Design review of the part built by this model. Coordinates are the model's own, in mm. A direction names the side the tool comes from. Give positions to 0.01 mm unless a question says otherwise; leave off trailing zeros. Write each loop counter-clockwise with the first axis right and the second up, starting at its lowest first coordinate (ties: lowest second). Pieces come first, ordered by that corner, then holes. Notation, with made-up numbers: M 39,-0.75 L 59,-0.75 A13 ccw 59,16.25 Z; hole C 41.25,76.5 d3. An arc over 180 degrees is marked long. Use one line per item in the form item = value. Start each with the question number.
from build123d import *

# Parameters (mm, degrees)
SKETCH1_R           = 22.45
SKETCH1_R_2         = 18.55
SKETCH1_R_3         = 6.11
SKETCH1_R_4         = 5.25
SKETCH1_R_5         = 3.075
BOSS_EXTRUDE1_DEPTH = 5.5
SKETCH1_3_R         = 22.45
SKETCH1_3_R_2       = 18.55
SKETCH1_3_R_3       = 6.11
BOSS_EXTRUDE2_DEPTH = 6
SKETCH1_4_R         = 22.45
SKETCH1_4_R_2       = 18.55
BOSS_EXTRUDE3_DEPTH = 17
BOSS_EXTRUDE4_DEPTH = 10
DRAFT1_ANGLE        = 45
BOSS_EXTRUDE5_DEPTH = 3
SKETCH4_R           = 3.075
BOSS_EXTRUDE6_DEPTH = 1.5
SKETCH3_R           = 1.5
SKETCH3_R_2         = 1.55
CUT_EXTRUDE1_DEPTH  = 11
CUT_EXTRUDE2_START  = -9.6
SKETCH3_4_R         = 1.5
CUT_EXTRUDE2_DEPTH  = 2.6
CUT_EXTRUDE3_START  = -8
SKETCH3_5_R         = 1.55
CUT_EXTRUDE3_DEPTH  = 2.5


with BuildPart() as part:
    # Sketch1 → Boss-Extrude1 (new body)
    with BuildSketch(Plane.ZY.offset(-4.58817912)):
        with BuildLine():
            Line((173.913255387, 21.29653024), (97.713255387, 21.29653024))
            Line((97.713255387, 21.29653024), (97.713255387, 24.29653024))
            Line((97.713255387, 24.29653024), (94.713255387, 24.29653024))
            Line((94.713255387, 24.29653024), (94.713255387, 18.29653024))
            ThreePointArc((94.713255387, 18.29653024), (95.445488434, 16.528763287), (97.213255387, 15.79653024))
            Line((97.213255387, 15.79653024), (102.52576333, 15.79653024))
            Line((102.52576333, 15.79653024), (102.52576333, -6.35346976))
            ThreePointArc((102.52576333, -6.35346976), (124.97576333, 16.09653024), (147.42576333, -6.35346976))
            Line((147.42576333, -6.35346976), (147.42576333, 13.29653024))
            Line((147.42576333, 13.29653024), (171.913255387, 13.29653024))
            ThreePointArc((171.913255387, 13.29653024), (175.448789293, 14.760996334), (176.913255387, 18.29653024))
            Line((176.913255387, 18.29653024), (176.913255387, 24.29653024))
            Line((176.913255387, 24.29653024), (173.913255387, 24.29653024))
            Line((173.913255387, 24.29653024), (173.913255387, 21.29653024))
        make_face()
        with BuildLine():
            ThreePointArc((124.97576333, -28.80346976), (109.101216092, -22.228016998), (102.52576333, -6.35346976))
            Line((102.52576333, -6.35346976), (102.52576333, -28.80346976))
            Line((102.52576333, -28.80346976), (124.97576333, -28.80346976))
        make_face()
        with Locations((124.97576333, -6.35346976)):
            Circle(SKETCH1_R)
        with Locations((124.97576333, -6.35346976)):
            Circle(SKETCH1_R_2, mode=Mode.SUBTRACT)
        with Locations((124.97576333, -6.35346976)):
            Circle(SKETCH1_R_2)
        with Locations((131.813255387, -4.853902367)):
            Circle(SKETCH1_R_3, mode=Mode.SUBTRACT)
        with Locations((131.813255387, -4.853902367)):
            Circle(SKETCH1_R_3)
        with Locations((131.813255387, -4.853902367)):
            Circle(SKETCH1_R_4, mode=Mode.SUBTRACT)
        with Locations((131.813255387, -4.853902367)):
            Circle(SKETCH1_R_4)
        with Locations((131.813255387, -4.853902367)):
            Circle(SKETCH1_R_5, mode=Mode.SUBTRACT)
        with BuildLine():
            Line((147.42576333, -28.80346976), (147.42576333, -6.35346976))
            ThreePointArc((147.42576333, -6.35346976), (140.850310568, -22.228016998), (124.97576333, -28.80346976))
            Line((124.97576333, -28.80346976), (147.42576333, -28.80346976))
        make_face()
    extrude(amount=BOSS_EXTRUDE1_DEPTH)

    # Sketch1<3> → Boss-Extrude2 (add)
    with BuildSketch(Plane.ZY.offset(-4.58817912)):
        with BuildLine():
            Line((173.913255387, 21.29653024), (97.713255387, 21.29653024))
            Line((97.713255387, 21.29653024), (97.713255387, 24.29653024))
            Line((97.713255387, 24.29653024), (94.713255387, 24.29653024))
            Line((94.713255387, 24.29653024), (94.713255387, 18.29653024))
            ThreePointArc((94.713255387, 18.29653024), (95.445488434, 16.528763287), (97.213255387, 15.79653024))
            Line((97.213255387, 15.79653024), (102.52576333, 15.79653024))
            Line((102.52576333, 15.79653024), (102.52576333, -6.35346976))
            ThreePointArc((102.52576333, -6.35346976), (124.97576333, 16.09653024), (147.42576333, -6.35346976))
            Line((147.42576333, -6.35346976), (147.42576333, 13.29653024))
            Line((147.42576333, 13.29653024), (171.913255387, 13.29653024))
            ThreePointArc((171.913255387, 13.29653024), (175.448789293, 14.760996334), (176.913255387, 18.29653024))
            Line((176.913255387, 18.29653024), (176.913255387, 24.29653024))
            Line((176.913255387, 24.29653024), (173.913255387, 24.29653024))
            Line((173.913255387, 24.29653024), (173.913255387, 21.29653024))
        make_face()
        with BuildLine():
            Line((147.42576333, -28.80346976), (147.42576333, -6.35346976))
            ThreePointArc((147.42576333, -6.35346976), (140.850310568, -22.228016998), (124.97576333, -28.80346976))
            Line((124.97576333, -28.80346976), (147.42576333, -28.80346976))
        make_face()
        with Locations((124.97576333, -6.35346976)):
            Circle(SKETCH1_3_R)
        with Locations((124.97576333, -6.35346976)):
            Circle(SKETCH1_3_R_2, mode=Mode.SUBTRACT)
        with Locations((124.97576333, -6.35346976)):
            Circle(SKETCH1_3_R_2)
        with Locations((131.813255387, -4.853902367)):
            Circle(SKETCH1_3_R_3, mode=Mode.SUBTRACT)
    extrude(amount=-BOSS_EXTRUDE2_DEPTH)

    # Sketch1<4> → Boss-Extrude3 (add)
    with BuildSketch(Plane.ZY.offset(-4.58817912)):
        with BuildLine():
            Line((173.913255387, 21.29653024), (97.713255387, 21.29653024))
            Line((97.713255387, 21.29653024), (97.713255387, 24.29653024))
            Line((97.713255387, 24.29653024), (94.713255387, 24.29653024))
            Line((94.713255387, 24.29653024), (94.713255387, 18.29653024))
            ThreePointArc((94.713255387, 18.29653024), (95.445488434, 16.528763287), (97.213255387, 15.79653024))
            Line((97.213255387, 15.79653024), (102.52576333, 15.79653024))
            Line((102.52576333, 15.79653024), (102.52576333, -6.35346976))
            ThreePointArc((102.52576333, -6.35346976), (124.97576333, 16.09653024), (147.42576333, -6.35346976))
            Line((147.42576333, -6.35346976), (147.42576333, 13.29653024))
            Line((147.42576333, 13.29653024), (171.913255387, 13.29653024))
            ThreePointArc((171.913255387, 13.29653024), (175.448789293, 14.760996334), (176.913255387, 18.29653024))
            Line((176.913255387, 18.29653024), (176.913255387, 24.29653024))
            Line((176.913255387, 24.29653024), (173.913255387, 24.29653024))
            Line((173.913255387, 24.29653024), (173.913255387, 21.29653024))
        make_face()
        with BuildLine():
            Line((147.42576333, -28.80346976), (147.42576333, -6.35346976))
            ThreePointArc((147.42576333, -6.35346976), (140.850310568, -22.228016998), (124.97576333, -28.80346976))
            Line((124.97576333, -28.80346976), (147.42576333, -28.80346976))
        make_face()
        with BuildLine():
            ThreePointArc((124.97576333, -28.80346976), (109.101216092, -22.228016998), (102.52576333, -6.35346976))
            Line((102.52576333, -6.35346976), (102.52576333, -28.80346976))
            Line((102.52576333, -28.80346976), (124.97576333, -28.80346976))
        make_face()
        with Locations((124.97576333, -6.35346976)):
            Circle(SKETCH1_4_R)
        with Locations((124.97576333, -6.35346976)):
            Circle(SKETCH1_4_R_2, mode=Mode.SUBTRACT)
    extrude(amount=-BOSS_EXTRUDE3_DEPTH)

    # Sketch2 → Boss-Extrude4 (add)
    with BuildSketch(Plane(origin=(21.58817912, 0, 0), x_dir=(0, 0, -1), z_dir=(1, 0, 0))):
        with BuildLine():
            Line((-151.941714705, 21.29653024), (-111.68479607, 21.29653024))
            ThreePointArc((-111.68479607, 21.29653024), (-131.813255387, 28.146097633), (-151.941714705, 21.29653024))
        make_face()
    extrude(amount=-BOSS_EXTRUDE4_DEPTH)

    # Draft1
    draft1_faces = [part.faces().sort_by_distance(p)[0] for p in [
        (11.58817912, 24.062292156, 131.813255387),
    ]]
    draft(draft1_faces, Plane(origin=(-98.771158707, 21.29653024, 0), x_dir=(1, 0, 0), z_dir=(0, 1, 0)), DRAFT1_ANGLE)

    # Sketch3<3> → Boss-Extrude5 (add)
    with BuildSketch(Plane(origin=(0, 21.29653024, 0), x_dir=(1, 0, 0), z_dir=(0, 1, 0))):
        with BuildLine():
            Line((-0.91182088, -173.913255387), (3.08817912, -173.913255387))
            ThreePointArc((3.08817912, -173.913255387), (0.526929425, -173.014817506), (-0.91182088, -170.713255387))
            Line((-0.91182088, -170.713255387), (-0.91182088, -173.913255387))
        make_face()
    extrude(amount=BOSS_EXTRUDE5_DEPTH)

    # Sketch4 → Boss-Extrude6 (add)
    with BuildSketch(Plane.ZY.offset(0.91182088)):
        with BuildLine():
            Line((97.713255387, 21.29653024), (97.713255387, 24.29653024))
            Line((97.713255387, 24.29653024), (94.713255387, 24.29653024))
            Line((94.713255387, 24.29653024), (94.713255387, 18.29653024))
            ThreePointArc((94.713255387, 18.29653024), (95.445488434, 16.528763287), (97.213255387, 15.79653024))
            Line((97.213255387, 15.79653024), (102.52576333, 15.79653024))
            Line((102.52576333, 15.79653024), (102.52576333, -28.80346976))
            Line((102.52576333, -28.80346976), (147.42576333, -28.80346976))
            Line((147.42576333, -28.80346976), (147.42576333, 13.29653024))
            Line((147.42576333, 13.29653024), (171.913255387, 13.29653024))
            ThreePointArc((171.913255387, 13.29653024), (175.448789293, 14.760996334), (176.913255387, 18.29653024))
            Line((176.913255387, 18.29653024), (176.913255387, 24.29653024))
            Line((176.913255387, 24.29653024), (170.713255387, 24.29653024))
            Line((170.713255387, 24.29653024), (170.713255387, 21.29653024))
            Line((170.713255387, 21.29653024), (155.075991135, 21.29653024))
            Line((155.075991135, 21.29653024), (108.550519639, 21.29653024))
            Line((108.550519639, 21.29653024), (97.713255387, 21.29653024))
        make_face()
        with Locations((131.813255387, -4.853902367)):
            Circle(SKETCH4_R, mode=Mode.SUBTRACT)
        with BuildLine():
            Line((112.44182594, 24.29653024), (97.713255387, 24.29653024))
            Line((97.713255387, 24.29653024), (97.713255387, 21.29653024))
            Line((97.713255387, 21.29653024), (108.550519639, 21.29653024))
            ThreePointArc((108.550519639, 21.29653024), (110.443463379, 22.864899727), (112.44182594, 24.29653024))
        make_face()
        with BuildLine():
            ThreePointArc((151.184684835, 24.29653024), (153.183047396, 22.864899727), (155.075991135, 21.29653024))
            Line((155.075991135, 21.29653024), (170.713255387, 21.29653024))
            Line((170.713255387, 21.29653024), (170.713255387, 24.29653024))
            Line((170.713255387, 24.29653024), (151.184684835, 24.29653024))
        make_face()
    extrude(amount=BOSS_EXTRUDE6_DEPTH)

    # Sketch3 → Cut-Extrude1 (cut)
    with BuildSketch(Plane(origin=(0, 21.29653024, 0), x_dir=(1, 0, 0), z_dir=(0, 1, 0))):
        with Locations(Location((2.879075654, -104.850755387, 0), (0, 0, 180))):
            Circle(SKETCH3_R)
        with Locations(Location((10.297282585, -104.850755387, 0), (0, 0, 180))):
            Circle(SKETCH3_R)
        with Locations(Location((3.11317912, -163.38083505, 0), (0, 0, 180))):
            Circle(SKETCH3_R_2)
    extrude(amount=-CUT_EXTRUDE1_DEPTH, mode=Mode.SUBTRACT)

    # Sketch3<4> → Cut-Extrude2 (cut)
    with BuildSketch(Plane(origin=(0, 21.29653024, 0), x_dir=(1, 0, 0), z_dir=(0, 1, 0)).offset(CUT_EXTRUDE2_START)):
        Polygon((7.447282585, -106.496203654), (10.297282585, -108.141651922), (13.147282585, -106.496203654), (13.147282585, -103.20530712), (11.970278215, -102.52576333), (8.624286956, -102.52576333), (7.447282585, -103.20530712), align=None)
        with Locations(Location((10.297282585, -104.850755387, 0), (0, 0, 180))):
            Circle(SKETCH3_4_R, mode=Mode.SUBTRACT)
        Polygon((11.970278215, -102.52576333), (13.147282585, -103.20530712), (13.147282585, -102.52576333), align=None)
        Polygon((7.447282585, -102.52576333), (7.447282585, -103.20530712), (8.624286956, -102.52576333), align=None)
        Polygon((0.029075654, -106.496203654), (2.879075654, -108.141651922), (5.729075654, -106.496203654), (5.729075654, -103.20530712), (4.552071284, -102.52576333), (1.206080025, -102.52576333), (0.029075654, -103.20530712), align=None)
        with Locations(Location((2.879075654, -104.850755387, 0), (0, 0, 180))):
            Circle(SKETCH3_4_R, mode=Mode.SUBTRACT)
        Polygon((4.552071284, -102.52576333), (5.729075654, -103.20530712), (5.729075654, -102.52576333), align=None)
        Polygon((0.029075654, -102.52576333), (0.029075654, -103.20530712), (1.206080025, -102.52576333), align=None)
    extrude(amount=CUT_EXTRUDE2_DEPTH, mode=Mode.SUBTRACT)

    # Sketch3<5> → Cut-Extrude3 (cut)
    with BuildSketch(Plane(origin=(0, 21.29653024, 0), x_dir=(1, 0, 0), z_dir=(0, 1, 0)).offset(CUT_EXTRUDE3_START)):
        Polygon((4.758627387, -160.53083505), (1.467730853, -160.53083505), (-0.177717415, -163.38083505), (1.467730853, -166.23083505), (4.758627387, -166.23083505), (6.404075654, -163.38083505), align=None)
        with Locations(Location((3.11317912, -163.38083505, 0), (0, 0, 180))):
            Circle(SKETCH3_5_R, mode=Mode.SUBTRACT)
    extrude(amount=CUT_EXTRUDE3_DEPTH, mode=Mode.SUBTRACT)


solid = part.part
1. We need section B-B (z = 168.5). State the section outline as (x, y) points.
2. Clearance check with flat-ended pins moving along their axes: pin 1 Ø2.5 at (x, z) = (9.5, 105.5) entering from +Y; pin 2 Ø2 at (x, y) = (17.5, -4.5) entering from -Z; pin 3 Ø18.5 at (y, z) = (-4.5, 123.5) entering from +X; pin 4 Ø2.5 at (y, z) = (22.5, 165.5) entering from +X. State where each tip first meets the part, or that it passes through.
3. To check wall thickness, follow L1, parallel to Y at x = 8.5, z = 103.5; L2, parallel to X at y = 6, z = 128; L3, parallel to X at y = 24, z = 143.5. State the ranges of each line that lie inside material, in increasing order.
4. We need section C-C (y = -15). State the section outline as (x, z) points.
5. Draft analysis for pull direction X (two halves, no side actions). For faces 1 (the flat face through (-0.912, 23, 103)), 2 (the flat face through (10, -28.803, 125)), 3 (the flat face through (3, 15, 166.231)), state which applies: pulls with the +X half, pulls with the -X half, needs draft (parallel to the pull), parting line crosses it, or undercut.
6. For faces 4 (the flat face through (5.57, 14.529, 164.826)), 5 (the flat face through (3, 10.297, 105)), 6 (the flat face through (10, 15.797, 100)), 7 (the flat face through (4.284, 12.978, 107.33)), 8 (the flat face through (10.588, -6, 125)), list the 3-axis set-ups (+Z, -Z, +X, -X, +Y, -Y) from which the entire face can be reached by the end or side of a thin tool; tool diameter is ignored.
7. We need section D-D (y = -0.5). State the section outline as (x, z) points, and give its area (3 significant figures).
8. We need section A-A (x = 17.5). State the section outline as (y, z) points, and give its area (3 significant figures).
Answer block:
q1.outline = M -2.41,13.3 L 21.59,13.3 L 21.59,21.3 L -0.91,21.3 L -0.91,24.3 L -2.41,24.3 Z
q2.pin_1 = 21.3
q2.pin_2 = 102.53
q2.pin_3 = 10.59
q2.pin_4 = 21.59
q3.L1 = -28.8 to 11.7, 14.3 to 21.3
q3.L2 = -2.41 to 10.59
q3.L3 = 14.29 to 21.59
q4.outline = M -2.41,102.53 L 21.59,102.53 L 21.59,108.56 L 10.59,108.56 L 10.59,141.39 L 21.59,141.39 L 21.59,147.43 L -2.41,147.43 Z
q5.face_1 = pulls with the +X half
q5.face_2 = needs draft
q5.face_3 = undercut
q6.face_4 = -Y
q6.face_5 = +Y
q6.face_6 = -Z, +X, -X, -Y
q6.face_7 = -Z
q6.face_8 = +X
q7.outline = M -2.41,102.53 L 21.59,102.53 L 21.59,107.37 L 10.59,107.37 L 10.59,127.53 L 4.59,127.53 L 4.59,136.1 L 10.59,136.1 L 10.59,142.58 L 21.59,142.58 L 21.59,147.43 L -2.41,147.43 Z
q7.area = 639 mm^2
q8.outline = M -28.8,102.53 L 15.8,102.53 L 15.8,97.21 A2.5 ccw 18.3,94.71 L 24.3,94.71 L 24.3,97.71 L 21.3,97.71 L 21.3,111.68 A33 ccw 27.21,124 L 27.21,139.62 A33 ccw 21.3,151.94 L 21.3,173.91 L 24.3,173.91 L 24.3,176.91 L 18.3,176.91 A5 ccw 13.3,171.91 L 13.3,147.43 L -28.8,147.43 Z; hole C -6.35,124.98 d37.1
q8.area = 1,640 mm^2
